Geometry: final body of the model. Coordinates: model frame, mm. Face numbers are marked on the shaded views. Round coordinates to 2 decimals unless told otherwise and drop trailing zeros. Loops run counter-clockwise (first coordinate to the right, second up) from the corner with the lowest first, then second, coordinate; pieces in that order, holes last. Notation, with made-up numbers: M -12.75,-17.75 L 17.25,-17.75 A18 ccw 17.25,-0.75 Z; hole C 4,34.25 d5. An arc over 180 degrees is marked long. Answer as a JSON object with one key per item and string values.
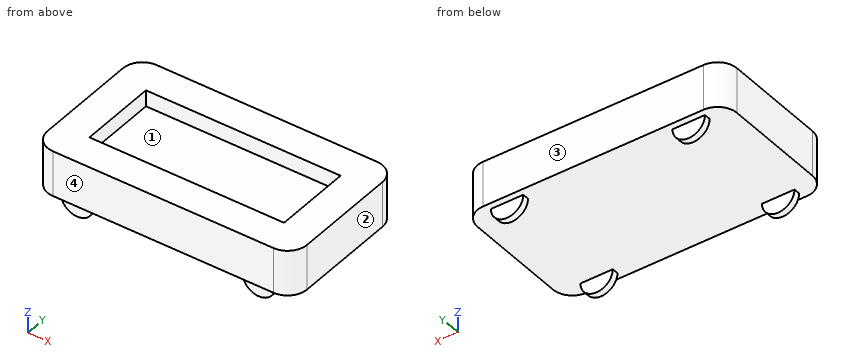
```python
from build123d import *

# Parameters (mm, degrees)
SKETCH1_W           = 40
SKETCH1_H           = 22
BOSS_EXTRUDE1_DEPTH = 7
FILLET1_R           = 3
SKETCH3_W           = 30
SKETCH3_H           = 12
CUT_EXTRUDE1_DEPTH  = 2.5
BOSS_EXTRUDE2_DEPTH = 1


with BuildPart() as part:
    # Sketch1 → Boss-Extrude1 (new body)
    with BuildSketch(Plane.XY):
        with Locations((20, 11)):
            Rectangle(SKETCH1_W, SKETCH1_H)
    extrude(amount=BOSS_EXTRUDE1_DEPTH)

    # Fillet1
    fillet1_edges = [part.edges().sort_by_distance(p)[0] for p in [
        (0, 22, 3.5),
        (40, 22, 3.5),
        (40, 0, 3.5),
        (0, 0, 3.5),
    ]]
    fillet(fillet1_edges, radius=FILLET1_R)

    # Sketch3 → Cut-Extrude1 (cut)
    with BuildSketch(Plane.XY.offset(7)):
        with Locations((20, 11)):
            Rectangle(SKETCH3_W, SKETCH3_H)
    extrude(amount=-CUT_EXTRUDE1_DEPTH, mode=Mode.SUBTRACT)

    # Sketch4 → Boss-Extrude2 (add)
    with BuildSketch(Plane(origin=(0, 21, 0), x_dir=(1, 0, 0), z_dir=(0, 1, 0))):
        with BuildLine():
            ThreePointArc((31.5, 0), (34, -2.5), (36.5, 0))
            Line((36.5, 0), (31.5, 0))
        make_face()
        with BuildLine():
            Line((31.5, 0), (36.5, 0))
            ThreePointArc((36.5, 0), (34, 2.5), (31.5, 0))
        make_face()
        with BuildLine():
            ThreePointArc((3.5, 0), (6, -2.5), (8.5, 0))
            Line((8.5, 0), (3.5, 0))
        make_face()
        with BuildLine():
            Line((3.5, 0), (8.5, 0))
            ThreePointArc((8.5, 0), (6, 2.5), (3.5, 0))
        make_face()
    boss_extrude2 = extrude(amount=-BOSS_EXTRUDE2_DEPTH)

    # Mirror1: Boss-Extrude2 across plane
    add(boss_extrude2.mirror(Plane(origin=(0, 11, 0), x_dir=(0, 0, 1), z_dir=(0, -1, 0))))


solid = part.part
```
1) Cut plane A-A on z = -1.5. Return the cut outline in (x, y).
Geometry results:
{"outline": "M 4,1 L 8,1 L 8,2 L 4,2 Z; M 4,20 L 8,20 L 8,21 L 4,21 Z; M 32,1 L 36,1 L 36,2 L 32,2 Z; M 32,20 L 36,20 L 36,21 L 32,21 Z"}
2) Cut plane D-D on y = 9. Return the cut outline in (x, z), and give its area (3 significant figures).
Geometry results:
{"outline": "M 0,0 L 40,0 L 40,7 L 35,7 L 35,4.5 L 5,4.5 L 5,7 L 0,7 Z", "area": "205 mm2"}
3) Line query: probe 1 along Y at (x, z) = (6, -1.75); probe 2 along Z at (x, y) = (31, 14); probe 3 along Z at (x, y) = (11.5, 20.25). Output: solid intervals per line, ascending.
Geometry results:
{"probe 1": "1 to 2, 20 to 21", "probe 2": "0 to 4.5", "probe 3": "0 to 7"}
4) Pull-direction query (Y, two-part tool) for the marked faces 1, 2, 3 and 4; classes: +Y half, -Y half, draft (parallel to the pull), parting line (faces both ways), or undercut.
Geometry results:
{"face 1": "undercut", "face 2": "draft", "face 3": "+Y half", "face 4": "-Y half"}
5) Cut plane B-B on z = 5.25. Return the cut outline in (x, y).
Geometry results:
{"outline": "M 0,3 A3 ccw 3,0 L 37,0 A3 ccw 40,3 L 40,19 A3 ccw 37,22 L 3,22 A3 ccw 0,19 Z; hole M 5,5 L 35,5 L 35,17 L 5,17 Z"}
6) Cut plane C-C on x = 4. Return the cut outline in (y, z), and give its area (3 significant figures).
Geometry results:
{"outline": "M 0,0 L 1,0 L 1,-1.5 L 2,-1.5 L 2,0 L 20,0 L 20,-1.5 L 21,-1.5 L 21,0 L 22,0 L 22,7 L 0,7 Z", "area": "157 mm2"}
7) First-contact query: pin 1 (0.8 mm diameter, centred on x = 6, z = -2, fed in from +Y); pin 2 (13 mm diameter, centred on x = 16.5, y = 8.5, fed in from +Z); pin 3 (0.8 mm diameter, centred on x = 35, z = -1, fed in from -Y); pin 4 (3 mm diameter, centred on x = 28.5, y = 9.5, fed in from -Z). Flat tips, straight axial feed; report the tip coordinate or a pass-through.
Geometry results:
{"pin 1": "y = 21", "pin 2": "z = 7", "pin 3": "y = 1", "pin 4": "z = 0"}
